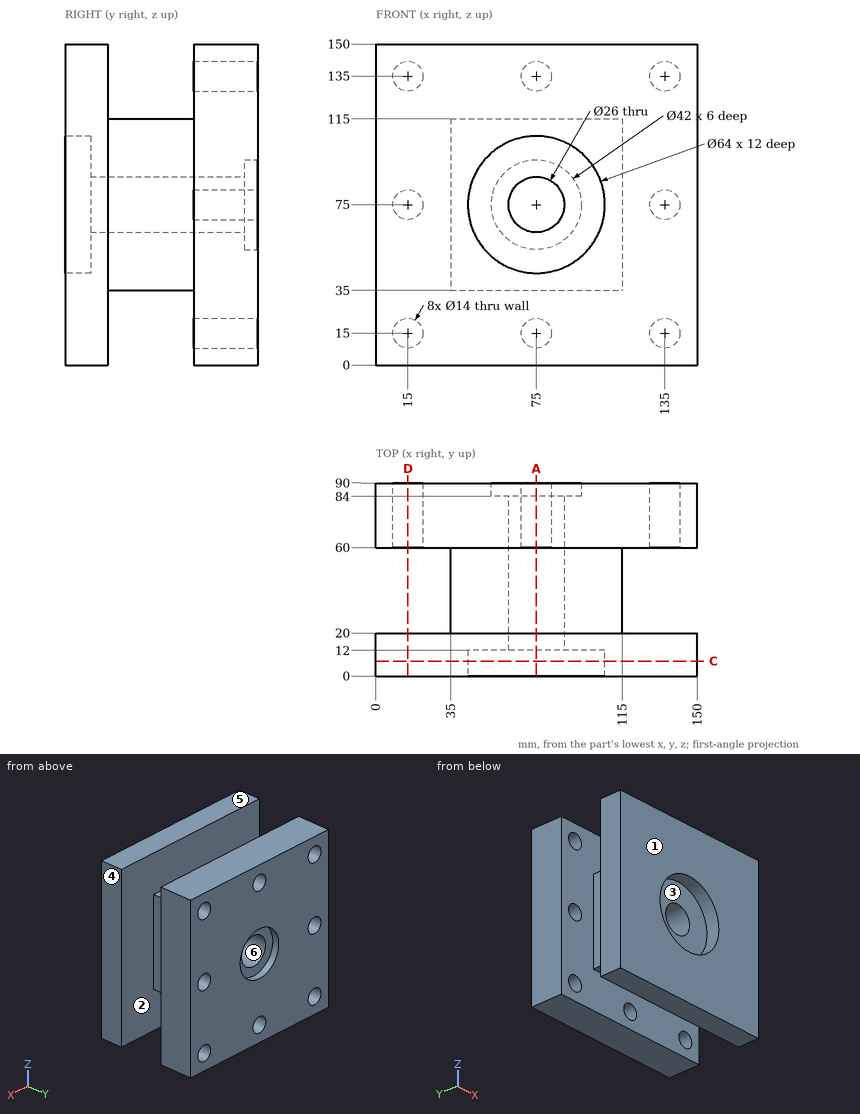
Source: three-view drawing plus pictorial views. Frame: mm from the lowest corner of the part. A direction names the side the tool comes from. Round coordinates to 2 decimals unless told otherwise and drop trailing zeros. Order: outer loops, then holes, each group sorted by start corner. A loop starts at its lowest first (then second) coordinate and runs counter-clockwise, first axis right, second up. Notation, with made-up numbers: (83.25, 35.5) -> (119.25, 35.5) arc R36 ccw to (119.25, 74.5) -> close; hole circle Ø7 at (5, -38.5). An arc over 180 degrees is marked (long way). Use one line per item in the form item = value. Start each with the question number.
1. Draft query along X for the marked faces 4, 5 and 6. Return one class per face: pulls with the +X half, pulls with the -X half, needs draft (parallel to the pull), parting line crosses it, or undercut.
2. Cut plane A-A (x = 75). Count the separate pieces of the cut face and the enclosed holes in it, then the cut area to 3 significant figures.
3. Line query: probe 1 along Z at (x, y) = (15, 68.75); probe 2 along Z at (x, y) = (75, 87); probe 3 along Y at (x, z) = (88.5, 21.5). Output: solid intervals per line, ascending.
4. Cut plane C-C (y = 7). Return the cut outline in (x, z), then the cut area to 3 significant figures.
5. Pin query (flat end, axial travel): pin 1 Ø6 at (y, z) = (28.5, 84) entering from -X; pin 2 Ø12 at (x, y) = (65.5, 43) entering from +Z; pin 3 Ø3 at (y, z) = (25.5, 95) entering from +X. Return the tip coordinate at first contact, or that it passes through.
6. Cut plane D-D (x = 15). Return the cut outline in (y, z).
7. Reachability of the marked faces 1, 2 and 3 from +Z, -Z, +X, -X, +Y, -Y: full face, straight path, thin tool, end or side. Return the list, or none.
Solution:
q1.face_4 = pulls with the +X half
q1.face_5 = needs draft
q1.face_6 = undercut
q2.separate_pieces = 4
q2.enclosed_holes = 0
q2.area = 6,970 mm^2
q3.probe_1 = 0 to 8, 22 to 68, 82 to 128, 142 to 150
q3.probe_2 = 0 to 8, 22 to 54, 96 to 128, 142 to 150
q3.probe_3 = 0 to 20, 60 to 90
q4.outline = (0, 0) -> (150, 0) -> (150, 150) -> (0, 150) -> close; hole circle Ø64 at (75, 75)
q4.area = 19,300 mm^2
q5.pin_1 = 35
q5.pin_2 = 115
q5.pin_3 = 115
q6.outline = (0, 0) -> (20, 0) -> (20, 150) -> (0, 150) -> close; (60, 0) -> (90, 0) -> (90, 8) -> (60, 8) -> close; (60, 22) -> (90, 22) -> (90, 68) -> (60, 68) -> close; (60, 82) -> (90, 82) -> (90, 128) -> (60, 128) -> close; (60, 142) -> (90, 142) -> (90, 150) -> (60, 150) -> close
q7.face_1 = +Z, -Z, +X, -X, -Y
q7.face_2 = none
q7.face_3 = -Y
